For this review, use the dimensioned drawing (mm, ordinates from the lowest corner) and the shaded views. A direction names the side the tool comes from. Round coordinates to 2 decimals unless told otherwise and drop trailing zeros. Order: outer loops, then holes, each group sorted by start corner. A loop starts at its lowest first (then second) coordinate and runs counter-clockwise, first axis right, second up. Notation, with made-up numbers: M 79.25,27.25 L 103.25,27.25 A32 ccw 103.25,63.25 Z; hole C 4,52.25 d2. An arc over 180 degrees is marked long. Put each result on its own line as item: value.
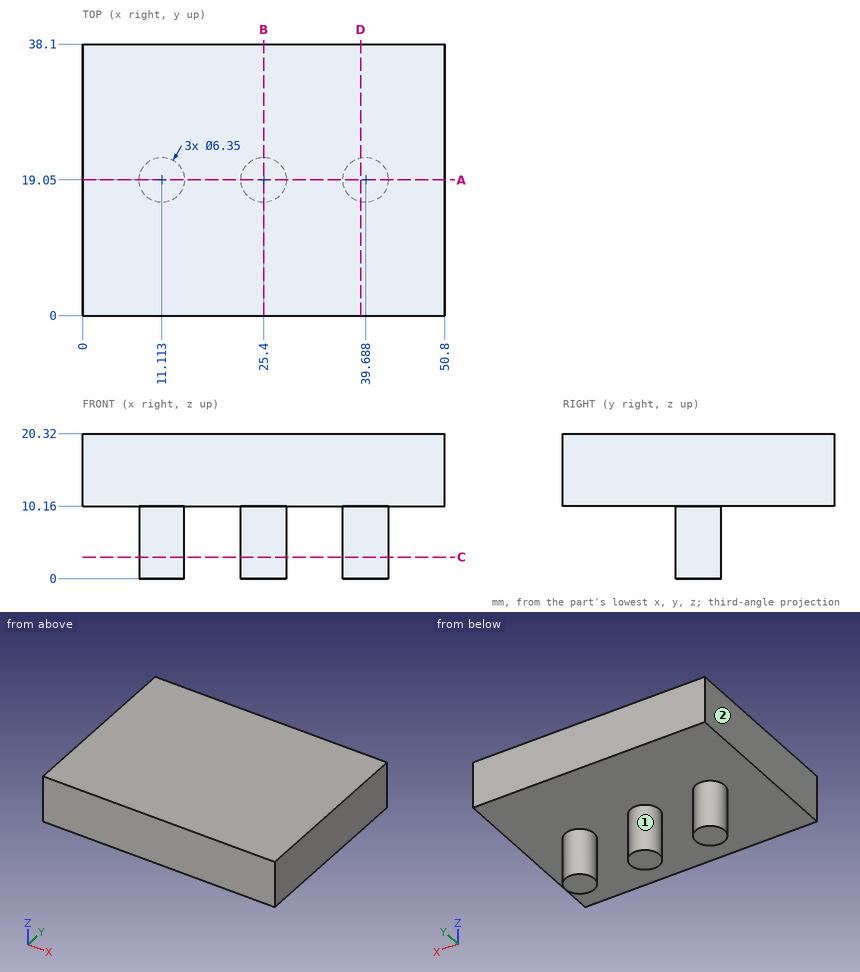
(1) Insertion check: pin 1 Ø12 at (x, y) = (8.5, 29) entering from -Z; pin 2 Ø1 at (x, z) = (14, 8.5) entering from -Y (1 decimal). Each pin has a flat end and moves straight along its axis. Give the tip position at first contact, or say it passes through.
A:
pin 1: stops at z = 10.16
pin 2: stops at y = 17
(2) Add section B-B on x = 25.4. Give the boundary of the cut face in (y, z) (1 decimal).
A:
outline: M 0,10.2 L 15.9,10.2 L 15.9,0 L 22.2,0 L 22.2,10.2 L 38.1,10.2 L 38.1,20.3 L 0,20.3 Z
(3) Add section C-C on z = 3. State how many separate pieces and enclosed holes the cut face has.
A:
separate pieces: 3
enclosed holes: 0
(4) To check wall thickness, follow L1, parallel to Z at x = 20, y = 20.5. State the ranges of the line that lie inside material, in increasing order.
A:
L1: z = 10.16 to 20.32
(5) Add section A-A on y = 19.05. Give the boundary of the cut face in (x, z) (1 decimal).
A:
outline: M 0,10.2 L 7.9,10.2 L 7.9,0 L 14.3,0 L 14.3,10.2 L 22.2,10.2 L 22.2,0 L 28.6,0 L 28.6,10.2 L 36.5,10.2 L 36.5,0 L 42.9,0 L 42.9,10.2 L 50.8,10.2 L 50.8,20.3 L 0,20.3 Z
(6) Add section D-D on x = 39. Give the boundary of the cut face in (y, z), then the cut area to 3 significant figures.
A:
outline: M 0,10.16 L 15.95,10.16 L 15.95,0 L 22.15,0 L 22.15,10.16 L 38.1,10.16 L 38.1,20.32 L 0,20.32 Z
area: 450 mm2
(7) For the marked faces 1 and 2, list the 3-axis set-ups (+Z, -Z, +X, -X, +Y, -Y) from which the entire face can be reached by the end or side of a thin tool; tool diameter is ignored.
A:
face 1: -Z
face 2: +Z, -Z, -X, +Y, -Y
